```python
from build123d import *

# Parameters (mm, degrees)
BRKT_3_4_BOSS_EXTRUDE1_START = -60
BRKT_3_4_BOSS_EXTRUDE1_DEPTH = 120
BOSS_EXTRUDE1_DEPTH          = 8


# Read off the part's stored shape, not the designer's step: <BRKT_3_4>-<Boss-Extrude1>
with BuildPart() as part:
    # <BRKT_3_4>-<Boss-Extrude1> outline → <BRKT_3_4>-<Boss-Extrude1> (new body)
    with BuildSketch(Plane.XY.offset(BRKT_3_4_BOSS_EXTRUDE1_START)):
        Polygon((0, 0), (0, -70), (8, -70), (8, -4.452742878), (63.708134873, 30.087764141), (59.492488509, 36.886905685), align=None)
    extrude(amount=BRKT_3_4_BOSS_EXTRUDE1_DEPTH)

    # Sketch1 → Boss-Extrude1 (add)
    with BuildSketch(Plane(origin=(0, 0, -60), x_dir=(-1, 0, 0), z_dir=(0, 0, -1))):
        Polygon((-63.708134873, 30.087764141), (-47.899461008, 55.58454493), (22, 12.245042915), (22, -70), (0, -70), (-8, -70), (-8, -4.452742878), align=None)
    extrude(amount=BOSS_EXTRUDE1_DEPTH)


solid = part.part
```
Read the model definition and answer for the solid it produces. Units are mm, in the model's axes. A direction names the side the tool comes from. Coordinates: 2 decimals unless noted, no trailing zeros. Loops run counter-clockwise (first coordinate to the right, second up) from the corner with the lowest first, then second, coordinate; pieces in that order, holes last. Notation, with made-up numbers: (48, -8) - (55, -8) arc R24 ccw to (55, 3) - close; hole circle Ø8 at (24.5, 57.5). An arc over 180 degrees is marked (long way). Answer in a Markdown table with one row per item.
1. Find section B-B, the plane x = 51.5. Write down the section's boundary in (y, z), then the cut area to 3 significant figures.
Conclusion:
| item | result |
|---|---|
| outline | (22.52, -68) - (49.78, -68) - (49.78, -60) - (31.93, -60) - (31.93, 60) - (22.52, 60) - close |
| area | 1,350 mm² |
2. Straight lines are drawn through the part: line 1 (Z direction, x = 33, y = 30); line 2 (X direction, y = -38, z = 19); line 3 (Y direction, x = 35, z = 32). For each, find the intervals that lie inside material, in ascending order.
Conclusion:
| item | result |
|---|---|
| line 1 | z = -68 to -60 |
| line 2 | x = 0 to 8 |
| line 3 | y = 12.29 to 21.7 |
3. Which of the six approach directions +Z, -Z, +X, -X, +Y, -Y give full straight-line access (tool end or side, diameter ignored) to faces 1 (the face through (0, -35, -1)), 2 (the face through (30.16, 18.7, -0.84)), 3 (the face through (10, 0, 60)), 4 (the face through (2, -70, -13)), 5 (the face through (8, -38, -3))?
Conclusion:
| item | result |
|---|---|
| face 1 | +Z, -X, +Y, -Y |
| face 2 | +Z, -X, +Y |
| face 3 | +Z, +X, -X, +Y, -Y |
| face 4 | +Z, -Z, +X, -X, -Y |
| face 5 | +Z, -Z, +X, -Y |
4. Find section C-C, the plane y = 40. Write down the section's boundary in (x, z), then the cut area to 3 significant figures.
Conclusion:
| item | result |
|---|---|
| outline | (22.76, -68) - (57.56, -68) - (57.56, -60) - (22.76, -60) - close |
| area | 278 mm² |
5. Find section A-A, the plane z = -46. Write down the section's boundary in (x, y).
Conclusion:
| item | result |
|---|---|
| outline | (0, -70) - (8, -70) - (8, -4.45) - (63.71, 30.09) - (59.49, 36.89) - (0, 0) - close |
6. Find section D-D, the plane x = -14.5. Write down the section's boundary in (y, z).
Conclusion:
| item | result |
|---|---|
| outline | (-70, -68) - (16.9, -68) - (16.9, -60) - (-70, -60) - close |
7. Given pin 1 (1.5 mm diameter, centred on y = -49, z = 41.5, fed in from +X); pin 2 (8 mm diameter, centred on x = 44.5, z = 29, fed in from +Y); pin 3 (8 mm diameter, centred on y = -17, z = -31, fed in from -X), each flat-ended and moving along its own axis, determine where each tip first touches the part or whether it passes through.
Conclusion:
| item | result |
|---|---|
| pin 1 | stops at x = 8 |
| pin 2 | stops at y = 30.07 |
| pin 3 | stops at x = 0 |
